The model under review builds one solid part; all positions refer to its coordinate system, in mm. A direction names the side the tool comes from. Give positions to 0.01 mm unless a question says otherwise; leave off trailing zeros. Order: outer loops, then holes, each group sorted by start corner. A loop starts at its lowest first (then second) coordinate and runs counter-clockwise, first axis right, second up. Notation, with made-up numbers: (15, 1.25) - (36, 1.25) arc R11 cw to (36, 5.25) - close; hole circle Ø1 at (18, -16). An arc over 180 degrees is marked (long way). Write item = value, one per line. Start each with the question number.
1. We need section D-D, the plane x = -32. Give the boundary of the cut face in (y, z).
2. Machinability: for faces 4 (the flat face through (-27, 15, -16)), 5 (the flat face through (-30, 14, -13)), 6 (the flat face through (-32, 16, -23.341)), 7 (the flat face through (-18, 0, -16)), 8 (the flat face through (-18, 6, -32.18)), which of the approach directions +Z, -Z, +X, -X, +Y, -Y give a long, thin tool a straight path to every point of the face, cutting with its end or side? Answer none if there is none.
3. We need section A-A, the plane y = 9.25. Give the boundary of the cut face in (x, z), and give its area (3 significant figures).
4. Mouldability with a two-part tool opening along Y and no side actions: class faces 1 (the cylindrical face through (-35.05, 8.38, -0.43)), 2 (the flat face through (-31, 17, -16)), 3 (the flat face through (-33, 8, -16)) as pulls with the +Y half, pulls with the -Y half, needs draft (parallel to the pull), parting line crosses it, or undercut.
5. For P1, Ø0.5, axis at x = -1.5, z = -23.5, coming from the +Y side; P2, Ø6, axis at x = -22, z = -14, coming from the +Y side; P3, Ø1.7, axis at x = -1.5, z = -28, coming from the +Y side, all flat-tipped, find the tip position at first contact; note any pin that passes through.
6. We need section B-B, the plane z = -27.68. Give the boundary of the cut face in (x, y).
7. We need section C-C, the plane z = -8.5. Give the boundary of the cut face in (x, y).
8. Wall thickness on probe 1 along Z at (x, y) = (-2.5, 14.4); probe 2 along X at (y, z) = (14.3, -4.5); probe 3 along X at (y, z) = (14.5, -27.68): over which ranges is each line inside the solid? List them lowest first.
Autodesk Inventor part; units mm, degrees
ref_plane "YZ Plane" through (0, 0, 0) normal (1, 0, 0) x (0, 1, 0)
ref_plane "XZ Plane" through (0, 0, 0) normal (0, 1, 0) x (-1, 0, 0)
ref_plane "XY Plane" through (0, 0, 0) normal (0, 0, 1) x (1, 0, 0)
sketch "Sketch1" plane through (0, 0, 0) normal (0, 1, 0) x (-1, 0, 0)
  line L0 (0, 0) -> (35.5, 0)
  line L1 (35.5, 0) -> (35.5, -32.18)
  line L2 (35.5, -32.18) -> (0, -32.18)
  line L3 (0, -32.18) -> (0, 0)
  line L4 (33, -2.5) -> (2.5, -2.5)
  line L5 (2.5, -2.5) -> (2.5, -29.68)
  line L6 (2.5, -29.68) -> (33, -29.68)
  line L7 (33, -29.68) -> (33, -2.5)
  dimension "d0" = 32.18
  dimension "d1" = 35.5
  dimension "d2" = 2.5
  dimension "d3" = 2.5
  dimension "d4" = 2.5
  dimension "d5" = 2.5
extrude "Extrusion1" add sketch "Sketch1" along normal blind 2 contours L0 L1 L2 L3 | L7 L6 L5 L4
extrude "Extrusion2" add sketch "Sketch1" along normal blind 14
sketch "Sketch2" plane through (0, 14, 0) normal (0, 1, 0) x (1, 0, 0)
  line L0 (-33, 2.5) -> (-33, 29.68)
  line L1 (-33, 29.68) -> (-2.5, 29.68)
  line L2 (-2.5, 29.68) -> (-2.5, 2.5)
  line L3 (-2.5, 2.5) -> (-33, 2.5)
  line L4 (-35.5, 0) -> (0, 0)
  line L5 (0, 0) -> (0, 32.18)
  line L6 (0, 32.18) -> (-35.5, 32.18)
  line L7 (-35.5, 32.18) -> (-35.5, 0)
  line L8 (-35.5, 0) -> (-35.5, 32.18)
  line L9 (0, 32.18) -> (-35.5, 32.18)
  line L10 (-35.5, 0) -> (-27, 0)
  line L11 (-27, 0) -> (-27, 32.18)
  line L12 (-27, 32.18) -> (-35.5, 32.18)
  line L13 (-35.5, 32.18) -> (-35.5, 0)
  dimension "d10" = 8.5
extrude "Extrusion3" add sketch "Sketch2" along normal blind 3 contours L3 L11 L4 L7 L6 L1 L0 | L0 L1 L11 L3
sketch "Sketch3" plane through (0, 17, 0) normal (0, 1, 0) x (1, 0, 0)
  line L0 (-35.5, 0) -> (-27, 0)
  line L1 (-27, 0) -> (-27, 32.18)
  line L2 (-27, 32.18) -> (-35.5, 32.18)
  line L3 (-35.5, 32.18) -> (-35.5, 0)
  line L4 (-34, 23.341) -> (-29, 23.341)
  line L5 (-29, 23.341) -> (-29, 30.341)
  line L6 (-29, 30.341) -> (-34, 30.341)
  line L7 (-34, 30.341) -> (-34, 23.341)
  point P0 (0, 0)
  dimension "d13" = 7
  dimension "d14" = 5
  dimension "d15" = 2
extrude "Extrusion4" cut sketch "Sketch3" against normal blind 3 contours L7 L6 L5 L4
sketch "Sketch4" plane through (0, 14, 0) normal (0, 1, 0) x (1, 0, 0)
  line L0 (-27, 32.18) -> (-27, 29.68)
  line L1 (-27, 29.68) -> (-2.5, 29.68)
  line L2 (-2.5, 29.68) -> (-2.5, 2.5)
  line L3 (-2.5, 2.5) -> (-27, 2.5)
  line L4 (-27, 2.5) -> (-27, 0)
  line L5 (-27, 0) -> (0, 0)
  line L6 (0, 0) -> (0, 32.18)
  line L7 (0, 32.18) -> (-27, 32.18)
  line L8 (0, 32.18) -> (0, 0)
  line L9 (0, 0) -> (-35.5, 0)
  line L10 (0, 32.18) -> (-5, 32.18)
  line L11 (-5, 32.18) -> (-5, 0)
  line L12 (-5, 0) -> (0, 0)
  line L13 (0, 0) -> (0, 32.18)
  dimension "d18" = 5
extrude "Extrusion5" add sketch "Sketch4" along normal blind 1 contours L7 L6 L5 L11 L3 L2 L1 | L1 L2 L3 L11
sketch "Sketch5" plane through (0, 15, 0) normal (0, 1, 0) x (1, 0, 0)
  line L0 (-5, 32.18) -> (-5, 0)
  line L1 (-5, 2.5) -> (-27, 2.5)
  line L2 (-5, 29.68) -> (-5, 2.5)
  circle A0 centre (-5, 16.5) radius 4
  line L3 (-2.5, 29.68) -> (-2.5, 2.5)
  circle A1 centre (-2.5, 27.68) radius 1.5
  circle A2 centre (-2.5, 23.68) radius 1.5
  circle A3 centre (-2.5, 8.5) radius 1.5
  circle A4 centre (-2.5, 4.5) radius 1.5
  line L4 (-5, 0) -> (0, 0)
  line L5 (0, 32.18) -> (-5, 32.18)
  dimension "d21" = 8
  dimension "d22" = 14
  dimension "d23" = 3
  dimension "d24" = 3
  dimension "d25" = 3
  dimension "d26" = 3
  dimension "d29" = 4.5
  dimension "d30" = 8.5
  dimension "d31" = 4.5
  dimension "d32" = 8.5
extrude "Extrusion6" cut sketch "Sketch5" against normal blind 1
fillet "Fillet1" radius 1.5 4 edges at (0, 7.5, -32.18) (-35.5, 8.5, -32.18) (-35.5, 8.5, 0) (0, 7.5, 0)
equation "\"d3\" = d2"
equation "\"d4\" = d2"
equation "\"d5\" = d2"
equation "\"d31\" = d29"
equation "\"d32\" = d30"
properties material "ABS Plastic"
Model answer:
q1.outline = (0, -32.18) - (17, -32.18) - (17, -30.34) - (14, -30.34) - (14, -29.68) - (2, -29.68) - (2, -2.5) - (14, -2.5) - (14, -23.34) - (17, -23.34) - (17, 0) - (0, 0) - close
q2.face_4 = +Z, -Z, +Y
q2.face_5 = none
q2.face_6 = +Y
q2.face_7 = +Z, -Z, +X, -X, -Y
q2.face_8 = -Z, +X, -X, +Y, -Y
q3.outline = (-35.5, -30.68) arc R1.5 ccw to (-34, -32.18) - (-1.5, -32.18) arc R1.5 ccw to (0, -30.68) - (0, -1.5) arc R1.5 ccw to (-1.5, 0) - (-34, 0) arc R1.5 ccw to (-35.5, -1.5) - close; hole (-33, -29.68) - (-2.5, -29.68) - (-2.5, -2.5) - (-33, -2.5) - close
q3.area = 311 mm2
q4.face_1 = needs draft
q4.face_2 = pulls with the +Y half
q4.face_3 = undercut
q5.P1 = 14
q5.P2 = 2
q5.P3 = 15
q6.outline = (-35.5, 0) - (0, 0) - (0, 15) - (-1, 15) - (-1, 14) - (-2.5, 14) - (-2.5, 2) - (-33, 2) - (-33, 14) - (-34, 14) - (-34, 17) - (-35.5, 17) - close; (-29, 14) - (-27, 14) - (-27, 17) - (-29, 17) - close; (-5, 14) - (-4, 14) - (-4, 15) - (-5, 15) - close
q7.outline = (-35.5, 0) - (0, 0) - (0, 15) - (-1, 15) - (-1, 14) - (-2.5, 14) - (-2.5, 2) - (-33, 2) - (-33, 14) - (-27, 14) - (-27, 17) - (-35.5, 17) - close; (-5, 14) - (-4, 14) - (-4, 15) - (-5, 15) - close
q8.probe_1 = -32.18 to -29.18, -26.18 to -25.18, -22.18 to -19.62, -13.38 to -10, -7 to -6, -3 to 0
q8.probe_2 = -35.5 to -27, -5 to -4, -1 to 0
q8.probe_3 = -35.5 to -34, -29 to -27, -5 to -4, -1 to 0
